Could you check a few things on this model? Use its own coordinates, in mm. A direction names the side the tool comes from. Give positions to 0.01 mm unless a question says otherwise; leave off trailing zeros. Write each loop counter-clockwise with the first axis right and the second up, starting at its lowest first coordinate (ties: lowest second). Pieces come first, ordered by that corner, then holes. Notation, with made-up numbers: (-12, -19) - (12, -19) arc R13 cw to (12, 2) - close; hole circle Ø5 at (72.5, 61). An arc over 180 degrees is marked (long way). Answer in a Markdown table with one row per item.
from build123d import *

# Parameters (mm, degrees)
RESSALTO_EXTRUS_O1_DEPTH = 5
ESBO_O2_R                = 1.5
CORTE_EXTRUS_O1_DEPTH    = 5
FILETE1_R                = 10
CORTE_EXTRUS_O2_DEPTH    = 5
ESBO_O4_R                = 1.5
CORTE_EXTRUS_O3_DEPTH    = 5
FILETE2_R                = 5
CORTE_EXTRUS_O4_DEPTH    = 5


with BuildPart() as part:
    # Esboço1 → Ressalto-extrusão1 (new body)
    with BuildSketch(Plane.XY):
        with BuildLine():
            Line((-14.089663978, 13.135393664), (-14.089663978, 28.135393664))
            Line((-14.089663978, 28.135393664), (-34.089663978, 28.135393664))
            Line((-34.089663978, 28.135393664), (-34.089663978, 128.135393664))
            Line((-34.089663978, 128.135393664), (25.910336022, 128.135393664))
            Line((25.910336022, 128.135393664), (25.910336022, 28.135393664))
            Line((25.910336022, 28.135393664), (5.910336022, 28.135393664))
            Line((5.910336022, 28.135393664), (5.910336022, 13.135393664))
            ThreePointArc((5.910336022, 13.135393664), (-4.089663978, 3.135393664), (-14.089663978, 13.135393664))
        make_face()
    extrude(amount=RESSALTO_EXTRUS_O1_DEPTH)

    # Esboço2 → Corte-extrusão1 (cut)
    with BuildSketch(Plane.XY.offset(5)):
        with Locations((-4.089663978, 13.135393664)):
            Circle(ESBO_O2_R)
    extrude(amount=-CORTE_EXTRUS_O1_DEPTH, mode=Mode.SUBTRACT)

    # Filete1
    filete1_edges = [part.edges().sort_by_distance(p)[0] for p in [
        (5.910336022, 28.135393664, 2.5),
        (-14.089663978, 28.135393664, 2.5),
    ]]
    fillet(filete1_edges, radius=FILETE1_R)
    filete1_2_edges = [part.edges().sort_by_distance(p)[0] for p in [
        (25.910336022, 28.135393664, 2.5),
        (-34.089663978, 28.135393664, 2.5),
    ]]
    fillet(filete1_2_edges, radius=FILETE1_R - 0.0001)  # a hair under: the kernel refuses the full size

    # Esboço3 → Corte-extrusão2 (cut)
    with BuildSketch(Plane.XY.offset(5)):
        with BuildLine():
            ThreePointArc((-34.089663978, 38.135393664), (-27.631189305, 83.135393664), (-34.089663978, 128.135393664))
            Line((-34.089663978, 128.135393664), (-34.089663978, 38.135393664))
        make_face()
        with BuildLine():
            ThreePointArc((25.910336022, 38.135393664), (19.45186135, 83.135393664), (25.910336022, 128.135393664))
            Line((25.910336022, 128.135393664), (25.910336022, 38.135393664))
        make_face()
    extrude(amount=-CORTE_EXTRUS_O2_DEPTH, mode=Mode.SUBTRACT)

    # Esboço4 → Corte-extrusão3 (cut)
    with BuildSketch(Plane.XY.offset(5)):
        with Locations((-9.089663978, 123.135393664)):
            Circle(ESBO_O4_R)
        with Locations((0.910336022, 123.135393664)):
            Circle(ESBO_O4_R)
        with Locations((-9.089663978, 73.355393664)):
            Circle(ESBO_O4_R)
        with Locations((0.910336022, 73.355393664)):
            Circle(ESBO_O4_R)
    extrude(amount=-CORTE_EXTRUS_O3_DEPTH, mode=Mode.SUBTRACT)

    # Filete2
    filete2_edges = [part.edges().sort_by_distance(p)[0] for p in [
        (-34.089663978, 128.135393664, 2.5),
        (25.910336022, 128.135393664, 2.5),
    ]]
    fillet(filete2_edges, radius=FILETE2_R)

    # Esboço5 → Corte-extrusão4 (cut)
    with BuildSketch(Plane.XY.offset(5)):
        Polygon((-13.989663978, 118.545393664), (-6.089663978, 118.545393664), (-6.089663978, 126.045393664), (-2.089663978, 126.045393664), (-2.089663978, 118.545393664), (5.810336022, 118.545393664), (5.810336022, 77.945393664), (-2.089663978, 77.945393664), (-2.089663978, 70.445393664), (-6.089663978, 70.445393664), (-6.089663978, 77.945393664), (-13.989663978, 77.945393664), align=None)
    extrude(amount=-CORTE_EXTRUS_O4_DEPTH, mode=Mode.SUBTRACT)


solid = part.part
1) Will these pins go through, and if not, where does the flat tip stop? P1, Ø1.5, axis at y = 124, z = 2, coming from the +X side; P2, Ø2.5, axis at y = 14.5, z = 3, coming from the -X side; P3, Ø1.5, axis at y = 95.5, z = 2.5, coming from the -X side.
Check values:
| item | result |
|---|---|
| P1 | stops at x = 24.37 |
| P2 | stops at x = -14.09 |
| P3 | stops at x = -28.17 |
2) Imagine slicing it at C-C (x = -29). List the corners of the cut face in (y, z) for me.
Check values:
| item | result |
|---|---|
| outline | (29.42, 0) - (62.25, 0) - (62.25, 5) - (29.42, 5) - close; (104.02, 0) - (127.92, 0) - (127.92, 5) - (104.02, 5) - close |
3) Imagine slicing it at A-A (y = 105). List the corners of the cut face in (x, z) for me.
Check values:
| item | result |
|---|---|
| outline | (-29.13, 0) - (-13.99, 0) - (-13.99, 5) - (-29.13, 5) - close; (5.81, 0) - (20.95, 0) - (20.95, 5) - (5.81, 5) - close |
4) Imagine slicing it at D-D (y = 16.5). List the corners of the cut face in (x, z) for me.
Check values:
| item | result |
|---|---|
| outline | (-14.09, 0) - (5.91, 0) - (5.91, 5) - (-14.09, 5) - close |
5) If I drill on line 1 (Y direction, x = -4, z = 2.65); line 2 (Y direction, x = -11, z = 1.4); line 3 (Y direction, x = -8, z = 4.05), over which ranges is the centre line in solid material (lowest first)?
Check values:
| item | result |
|---|---|
| line 1 | y = 3.14 to 11.64, 14.63 to 70.45, 126.05 to 128.14 |
| line 2 | y = 5.91 to 77.95, 118.55 to 128.14 |
| line 3 | y = 3.93 to 72.32, 74.39 to 77.95, 118.55 to 122.1, 124.17 to 128.14 |
6) We'd pull the mould along X, two halves only. Please class faces 1 (the face through (-14.09, 16, 2)), 2 (the face through (-6.09, 122, 3)), 3 (the face through (-4, 67, 5)): +X half, -X half, draft (parallel to the pull), parting line (faces both ways), or undercut.
Check values:
| item | result |
|---|---|
| face 1 | -X half |
| face 2 | undercut |
| face 3 | draft |
7) On a 3-axis mill with a long thin cutter (end or side, diameter ignored), from which of +Z, -Z, +X, -X, +Y, -Y can I reach the whole of each face in a straight line? I mean faces 4 (the face through (-3.87, 3.138, 2.465)), 5 (the face through (2, 77.945, 3)). Say none if no direction works.
Check values:
| item | result |
|---|---|
| face 4 | +Z, -Z, -Y |
| face 5 | +Z, -Z |
8) Imagine slicing it at B-B (z = 0.95). State how many separate pieces and enclosed holes the cut face has, then the cut area to 3 significant figures.
Check values:
| item | result |
|---|---|
| separate pieces | 1 |
| enclosed holes | 6 |
| area | 4,760 mm2 |
